Read the model definition and answer for the solid it produces. Units are mm, in the model's axes. A direction names the side the tool comes from. Give positions to 0.01 mm unless a question says otherwise; leave off trailing zeros. Write each loop counter-clockwise with the first axis right and the second up, starting at its lowest first coordinate (ties: lowest second). Pieces come first, ordered by that corner, then holes.
```python
from build123d import *

# Parameters (mm, degrees)
CROQUIS1_W                   = 82
CROQUIS1_H                   = 78
CROQUIS1_R                   = 2.5
SALIENTE_EXTRUIR5_DEPTH      = 10
SALIENTE_EXTRUIR7_DEPTH      = 10
CORTAR_EXTRUIR_L_MINA1_START = -10
CORTAR_EXTRUIR_L_MINA1_DEPTH = 10


# Read off the part's stored shape, not the designer's step: Cortar-Extruir-Lámina1
with BuildPart() as part:
    # Croquis1 → Saliente-Extruir5 (new body)
    with BuildSketch(Plane.XY):
        Rectangle(CROQUIS1_W, CROQUIS1_H)
        with Locations((-33, 29.5)):
            Circle(CROQUIS1_R, mode=Mode.SUBTRACT)
        with Locations((33, 29.5)):
            Circle(CROQUIS1_R, mode=Mode.SUBTRACT)
        with Locations((33, -29.5)):
            Circle(CROQUIS1_R, mode=Mode.SUBTRACT)
        with Locations((-33, -29.5)):
            Circle(CROQUIS1_R, mode=Mode.SUBTRACT)
    extrude(amount=SALIENTE_EXTRUIR5_DEPTH)

    # Croquis6 → Saliente-Extruir7 (add, through all)
    with BuildSketch(Plane.XY.offset(10)):
        Polygon((-41, 17.857864376), (-41, 36), (-45.071067812, 31.928932188), (-45.071067812, 21.928932188), align=None)
        Polygon((45.071067812, 31.928932188), (41, 36), (41, 17.857864376), (45.071067812, 21.928932188), align=None)
        Polygon((-41, -39), (-41, -21.928932188), (-44.535533906, -25.464466094), (-44.535533906, -35.464466094), align=None)
        Polygon((44.535533906, -25.464466094), (41, -21.928932188), (41, -39), (44.535533906, -35.464466094), align=None)
        Polygon((-23.928932188, -39), (-41, -39), (-37.464466094, -42.535533906), (-27.464466094, -42.535533906), align=None)
        Polygon((37.464466094, -42.535533906), (41, -39), (23.928932188, -39), (27.464466094, -42.535533906), align=None)
    extrude(amount=-SALIENTE_EXTRUIR7_DEPTH)

    # Cortar-Extruir-Lámina1 outline → Cortar-Extruir-Lámina1 (cut)
    with BuildSketch(Plane.XY.offset(10).offset(CORTAR_EXTRUIR_L_MINA1_START)):
        Polygon((41, 39), (38, 39), (41, 36), align=None)
        Polygon((28, 39), (-28, 39), (-24.464466094, 35.464466094), (24.464466094, 35.464466094), align=None)
        Polygon((-41, 36), (-38, 39), (-41, 39), align=None)
    extrude(amount=CORTAR_EXTRUIR_L_MINA1_DEPTH, mode=Mode.SUBTRACT)


solid = part.part
```
Item 1: Determine the mould class of faces 6 (the flat face through (26, 37, 5)), 7 (the flat face through (-41, -2, 5)), 8 (the flat face through (-33, 39, 5)), 9 (the flat face through (44.536, -31, 5)) for opening direction X: pulls with the +X half, pulls with the -X half, needs draft (parallel to the pull), parting line crosses it, or undercut.
Result set:
face 6: undercut
face 7: pulls with the -X half
face 8: needs draft
face 9: pulls with the +X half
Item 2: Section D-D (y = 10) is taken. Write down the section's boundary in (x, z), and give its area (3 significant figures).
Result set:
outline: (-41, 0) - (41, 0) - (41, 10) - (-41, 10) - close
area: 820 mm2
Item 3: Each of these flat-tipped pins is pushed along its axis until it touches: pin 1 Ø4.5 at (x, y) = (-33, 29.5) entering from -Z; pin 2 Ø3 at (y, z) = (-31, 5.5) entering from +X; pin 3 Ø3 at (x, z) = (-10, 2.5) entering from +Y; pin 4 Ø5 at (x, z) = (11.5, 5) entering from -Y. Where does it stop, or does it pass through?
Result set:
pin 1: passes through
pin 2: stops at x = 44.54
pin 3: stops at y = 35.46
pin 4: stops at y = -39
Item 4: Section B-B (x = -33) is taken. Write down the section's boundary in (y, z), and give its area (3 significant figures).
Result set:
outline: (-42.54, 0) - (-32, 0) - (-32, 10) - (-42.54, 10) - close; (-27, 0) - (27, 0) - (27, 10) - (-27, 10) - close; (32, 0) - (39, 0) - (39, 10) - (32, 10) - close
area: 715 mm2
Item 5: Which of the six approach directions +Z, -Z, +X, -X, +Y, -Y give full straight-line access (tool end or side, diameter ignored) to faces 1 (the cylindrical face through (33, 32, 5)), 2 (the flat face through (42.79, -23.72, 5.07)), 3 (the flat face through (33, 39, 5)), 4 (the flat face through (0, -39, 5)), 5 (the flat face through (-42.74, -23.67, 5.07))?
Result set:
face 1: +Z, -Z
face 2: +Z, -Z, +X
face 3: +Z, -Z, +X, -X, +Y
face 4: +Z, -Z, -Y
face 5: +Z, -Z, -X
Item 6: Section A-A (y = 29.5) is taken. Write down the section's boundary in (x, z), and give its area (3 significant figures).
Result set:
outline: (-45.07, 0) - (-35.5, 0) - (-35.5, 10) - (-45.07, 10) - close; (-30.5, 0) - (30.5, 0) - (30.5, 10) - (-30.5, 10) - close; (35.5, 0) - (45.07, 0) - (45.07, 10) - (35.5, 10) - close
area: 801 mm2
Item 7: Find the intervals of material crossed by line 1 along X through (y, z) = (-29, 6.25); line 2 along Y through (x, z) = (33, 6); line 3 along X through (y, z) = (-27.5, 2.75), in increasing order.
Result set:
line 1: x = -44.54 to -35.45, -30.55 to 30.55, 35.45 to 44.54
line 2: y = -42.54 to -32, -27 to 27, 32 to 39
line 3: x = -44.54 to -34.5, -31.5 to 31.5, 34.5 to 44.54
Item 8: Section C-C (z = 5.25) is taken. Write down the section's boundary in (x, y).
Result set:
outline: (-45.07, 21.93) - (-41, 17.86) - (-41, -21.93) - (-44.54, -25.46) - (-44.54, -35.46) - (-37.46, -42.54) - (-27.46, -42.54) - (-23.93, -39) - (23.93, -39) - (27.46, -42.54) - (37.46, -42.54) - (44.54, -35.46) - (44.54, -25.46) - (41, -21.93) - (41, 17.86) - (45.07, 21.93) - (45.07, 31.93) - (38, 39) - (28, 39) - (24.46, 35.46) - (-24.46, 35.46) - (-28, 39) - (-38, 39) - (-45.07, 31.93) - close; hole circle Ø5 at (-33, -29.5); hole circle Ø5 at (-33, 29.5); hole circle Ø5 at (33, -29.5); hole circle Ø5 at (33, 29.5)
